```python
from build123d import *

# Parameters (mm, degrees)
SKETCH1_R           = 3.81
BOSS_EXTRUDE1_DEPTH = 12.7


with BuildPart() as part:
    # Sketch1 → Boss-Extrude1 (new body)
    with BuildSketch(Plane.XY):
        with BuildLine():
            Line((-21.102851537, -0.529390312), (-21.102851537, -5.609390312))
            Line((-21.102851537, -5.609390312), (16.997148463, -5.609390312))
            Line((16.997148463, -5.609390312), (16.997148463, -0.529390312))
            Line((16.997148463, -0.529390312), (4.297148463, -0.529390312))
            Line((4.297148463, -0.529390312), (4.297148463, 1.686095421))
            ThreePointArc((4.297148463, 1.686095421), (-2.052851537, 8.036095421), (-8.402851537, 1.686095421))
            Line((-8.402851537, 1.686095421), (-8.402851537, -0.529390312))
            Line((-8.402851537, -0.529390312), (-21.102851537, -0.529390312))
        make_face()
        with Locations((-2.052851537, 1.686095421)):
            Circle(SKETCH1_R, mode=Mode.SUBTRACT)
    extrude(amount=BOSS_EXTRUDE1_DEPTH)


solid = part.part
```
Work out the finished part from the listing and answer in its coordinate system (mm). A direction names the side the tool comes from. Coordinates: 2 decimals unless noted, no trailing zeros. Order: outer loops, then holes, each group sorted by start corner. A loop starts at its lowest first (then second) coordinate and runs counter-clockwise, first axis right, second up. Notation, with made-up numbers: (41, -38.5) - (100, -38.5) arc R23 cw to (100, -13.5) - close; hole circle Ø9 at (88.25, -27.5). An arc over 180 degrees is marked (long way). Answer as a JSON object with one key per item and string values.
1. Each of these flat-tipped pins is pushed along its axis until it touches: P1, Ø1.1, axis at y = 0.5, z = 6, coming from the +X side; P2, Ø1, axis at y = 6.5, z = 5, coming from the +X side; P3, Ø4, axis at x = 12, z = 6.5, coming from the +Y side. Where does it stop, or does it pass through?
Output values:
{"P1": "stops at x = 4.3", "P2": "stops at x = 2.61", "P3": "stops at y = -0.53"}
2. Consider line 1 (X direction, y = 1.5, z = 2); line 2 (Y direction, x = -14.5, z = 12); line 3 (X direction, y = 0, z = 12). Determine where each line is inside the solid, lowest interval first.
Output values:
{"line 1": "x = -8.4 to -5.86, 1.75 to 4.3", "line 2": "y = -5.61 to -0.53", "line 3": "x = -8.4 to -5.47, 1.36 to 4.3"}
3. Find section D-D on y = 0. Determine the outline of the cut face in (x, z), plus the area to 3 significant figures.
Output values:
{"outline": "(-8.4, 0) - (-5.47, 0) - (-5.47, 12.7) - (-8.4, 12.7) - close; (1.36, 0) - (4.3, 0) - (4.3, 12.7) - (1.36, 12.7) - close", "area": "74.5 mm²"}
4. Find section B-B on z = 5.5. Determine the outline of the cut face in (x, y).
Output values:
{"outline": "(-21.1, -5.61) - (17, -5.61) - (17, -0.53) - (4.3, -0.53) - (4.3, 1.69) arc R6.35 ccw to (-8.4, 1.69) - (-8.4, -0.53) - (-21.1, -0.53) - close; hole circle Ø7.62 at (-2.05, 1.69)"}
5. The mould has two halves that part along Y. Classify faces 4 (the face through (-1.913, 8.035, 6.261)), 5 (the face through (1.58, 2.83, 6.26)), 6 (the face through (-2, -3, 12.7)): +Y half, -Y half, draft (parallel to the pull), parting line (faces both ways), or undercut.
Output values:
{"face 4": "+Y half", "face 5": "undercut", "face 6": "draft"}
6. Find section C-C on x = 5. Determine the outline of the cut face in (y, z), plus the area to 3 significant figures.
Output values:
{"outline": "(-5.61, 0) - (-0.53, 0) - (-0.53, 12.7) - (-5.61, 12.7) - close", "area": "64.5 mm²"}
7. A tool of negligible diameter and unlimited length cuts with its end or side. For faces 1 (the face through (-2, -5.609, 6)), 2 (the face through (4.297, 1, 6)), 3 (the face through (-15, -0.529, 6)), from which of +Z, -Z, +X, -X, +Y, -Y can it reach the whole face along a straight path? Write none if from no direction.
Output values:
{"face 1": "+Z, -Z, +X, -X, -Y", "face 2": "+Z, -Z, +X, +Y", "face 3": "+Z, -Z, -X, +Y"}
8. Find section A-A on y = 4.75. Determine the outline of the cut face in (x, z).
Output values:
{"outline": "(-7.61, 0) - (-4.32, 0) - (-4.32, 12.7) - (-7.61, 12.7) - close; (0.21, 0) - (3.51, 0) - (3.51, 12.7) - (0.21, 12.7) - close"}
